Geometry check sheet. Reference: drawing and pictorial views, mm from the part's lowest x, y, z. Give positions to 0.01 mm unless a question says otherwise; leave off trailing zeros. Order: outer loops, then holes, each group sorted by start corner. A loop starts at its lowest first (then second) coordinate and runs counter-clockwise, first axis right, second up.
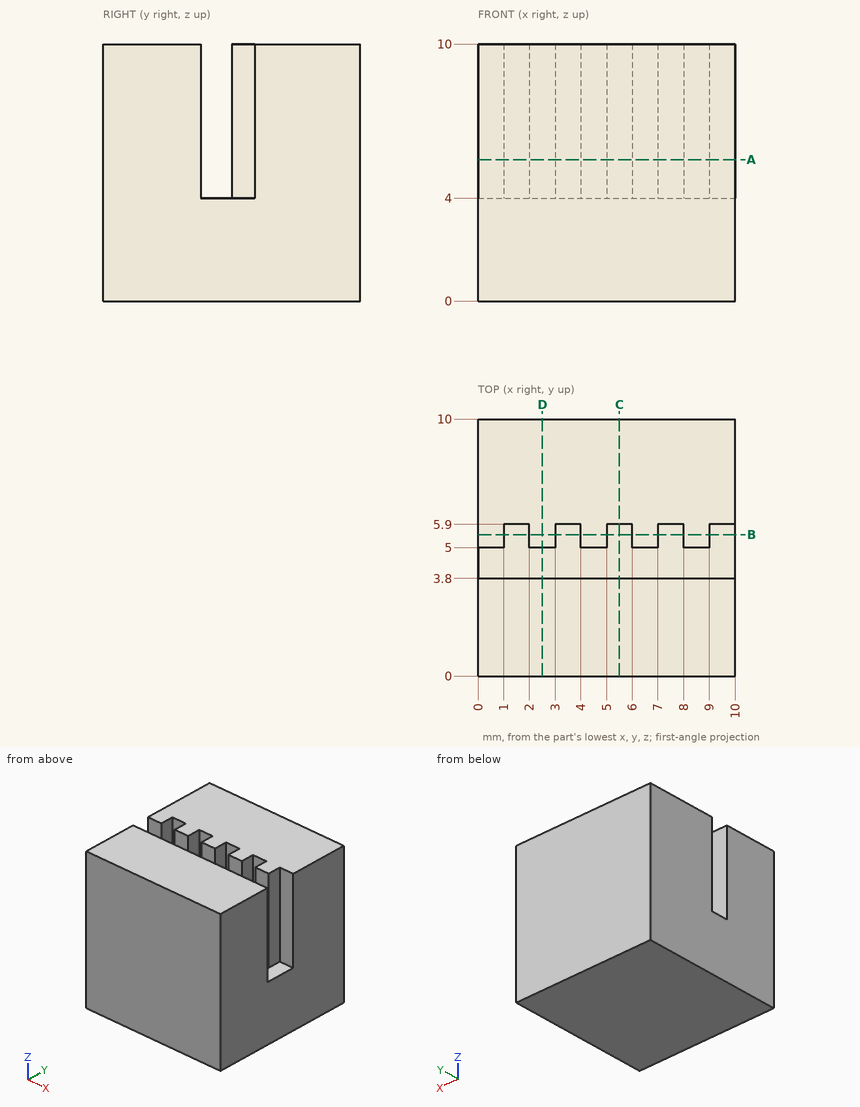
1) Section check B-B, the plane y = 5.5. Record the cut outline in (x, z), then the cut area to 3 significant figures.
Recorded:
outline: (0, 0) - (10, 0) - (10, 4) - (9, 4) - (9, 10) - (8, 10) - (8, 4) - (7, 4) - (7, 10) - (6, 10) - (6, 4) - (5, 4) - (5, 10) - (4, 10) - (4, 4) - (3, 4) - (3, 10) - (2, 10) - (2, 4) - (1, 4) - (1, 10) - (0, 10) - close
area: 70.0 mm2
2) Section check A-A, the plane z = 5.5. Record the cut outline in (x, y).
Recorded:
outline: (0, 0) - (10, 0) - (10, 3.8) - (0, 3.8) - close; (0, 5) - (1, 5) - (1, 5.9) - (2, 5.9) - (2, 5) - (3, 5) - (3, 5.9) - (4, 5.9) - (4, 5) - (5, 5) - (5, 5.9) - (6, 5.9) - (6, 5) - (7, 5) - (7, 5.9) - (8, 5.9) - (8, 5) - (9, 5) - (9, 5.9) - (10, 5.9) - (10, 10) - (0, 10) - close
3) Section check C-C, the plane x = 5.5. Record the cut outline in (y, z).
Recorded:
outline: (0, 0) - (10, 0) - (10, 10) - (5.9, 10) - (5.9, 4) - (3.8, 4) - (3.8, 10) - (0, 10) - close
4) Depth check by flat-ended pin: pin 1 Ø0.5 at (y, z) = (5, 7.5) entering from +X. Enter the tip coordinate at first touch or a pass-through.
Recorded:
pin 1: stops at x = 9
5) Section check D-D, the plane x = 2.5. Record the cut outline in (y, z).
Recorded:
outline: (0, 0) - (10, 0) - (10, 10) - (5, 10) - (5, 4) - (3.8, 4) - (3.8, 10) - (0, 10) - close
6) Material ranges on L1, parallel to Y at x = 8.5, z = 5.25; L2, parallel to Y at x = 7.75, z = 7.5; L3, parallel to Z at x = 5.5, y = 4.75, recorded low to high.
Recorded:
L1: y = 0 to 3.8, 5 to 10
L2: y = 0 to 3.8, 5.9 to 10
L3: z = 0 to 4
